Design review of the part built by this model. Coordinates are the model's own, in mm. A direction names the side the tool comes from. Coordinates: 2 decimals unless noted, no trailing zeros. Write each loop counter-clockwise with the first axis right and the second up, starting at its lowest first coordinate (ties: lowest second). Pieces come first, ordered by that corner, then holes. Notation, with made-up numbers: (-24, 32.25) - (7, 32.25) arc R5 cw to (7, 38.25) - close; hole circle Ø5 at (20.5, 20). An arc over 180 degrees is marked (long way). Answer as a JSON object with one key per item and string values.
```python
from build123d import *

# Parameters (mm, degrees)
SKETCH_2_W               = 50
SKETCH_2_H               = 30
SKETCH_2_W_2             = 48
SKETCH_2_H_2             = 28
EXTRUDE_1_DEPTH          = 150
SKETCH_3_R               = 1.525
CUT_EXTRUDE_1_DEPTH      = 10
PATTERN_LINEAR_1_COUNT   = 7
PATTERN_LINEAR_1_PITCH   = 30
SKETCH_4_R               = 1.525
CUT_EXTRUDE_2_DEPTH      = 10
PATTERN_LINEAR_2_COUNT   = 15
PATTERN_LINEAR_2_PITCH   = 20
CUT_EXTRUDE_3_DEPTH      = 10
PATTERN_LINEAR_3_COUNT   = 7
PATTERN_LINEAR_3_PITCH   = 40
SKETCH_6_R               = 4
CUT_EXTRUDE_4_DEPTH      = 10
PATTERN_LINEAR_4_COUNT   = 7
PATTERN_LINEAR_4_PITCH   = 30
SKETCH_7_R               = 1.525
CUT_EXTRUDE_5_DEPTH      = 90
SKETCH_8_R               = 1.525
CUT_EXTRUDE_6_DEPTH      = 10
SKETCH_10_R              = 1.525
CUT_EXTRUDE_7_DEPTH      = 51
SKETCH_12_R              = 1.525
CUT_EXTRUDE_9_DEPTH      = 1
CUT_EXTRUDE_9_DEPTH_BACK = 31
SKETCH_14_R              = 1.525
CUT_EXTRUDE_10_DEPTH     = 10


with BuildPart() as part:
    # 草图2 → 凸台-拉伸1 (new body, symmetric)
    with BuildSketch(Plane.XY):
        Rectangle(SKETCH_2_W, SKETCH_2_H)
        Rectangle(SKETCH_2_W_2, SKETCH_2_H_2, mode=Mode.SUBTRACT)
    extrude(amount=EXTRUDE_1_DEPTH, both=True)

    # 草图3 → 切除-拉伸1 (cut)
    with BuildSketch(Plane(origin=(25, 0, 0), x_dir=(0, 0, -1), z_dir=(1, 0, 0))):
        with Locations((-130, 5)):
            Circle(SKETCH_3_R)
    cut_extrude_1 = extrude(amount=-CUT_EXTRUDE_1_DEPTH, mode=Mode.SUBTRACT)

    # 阵列(线性)1: 切除-拉伸1 ×7
    with Locations(*[(0, 0, -i * PATTERN_LINEAR_1_PITCH) for i in range(1, PATTERN_LINEAR_1_COUNT)]):
        add(cut_extrude_1, mode=Mode.SUBTRACT)

    # 草图4 → 切除-拉伸2 (cut)
    with BuildSketch(Plane(origin=(0, 15, 0), x_dir=(1, 0, 0), z_dir=(0, 1, 0))):
        with Locations((-12, 140)):
            Circle(SKETCH_4_R)
        with Locations((12, 140)):
            Circle(SKETCH_4_R)
    cut_extrude_2 = extrude(amount=-CUT_EXTRUDE_2_DEPTH, mode=Mode.SUBTRACT)

    # 阵列(线性)2: 切除-拉伸2 ×15
    with Locations(*[(0, 0, i * PATTERN_LINEAR_2_PITCH) for i in range(1, PATTERN_LINEAR_2_COUNT)]):
        add(cut_extrude_2, mode=Mode.SUBTRACT)

    # 草图5 → 切除-拉伸3 (cut)
    with BuildSketch(Plane(origin=(0, -14, 0), x_dir=(1, 0, 0), z_dir=(0, 1, 0))):
        with BuildLine():
            Line((-17.5, -140), (-17.5, -120))
            ThreePointArc((-17.5, -120), (-12, -114.5), (-6.5, -120))
            Line((-6.5, -120), (-6.5, -140))
            ThreePointArc((-6.5, -140), (-12, -145.5), (-17.5, -140))
        make_face()
        with BuildLine():
            Line((17.5, -140), (17.5, -120))
            ThreePointArc((17.5, -120), (12, -114.5), (6.5, -120))
            Line((6.5, -120), (6.5, -140))
            ThreePointArc((6.5, -140), (12, -145.5), (17.5, -140))
        make_face()
    cut_extrude_3 = extrude(amount=-CUT_EXTRUDE_3_DEPTH, mode=Mode.SUBTRACT)

    # 阵列(线性)3: 切除-拉伸3 ×7
    with Locations(*[(0, 0, -i * PATTERN_LINEAR_3_PITCH) for i in range(1, PATTERN_LINEAR_3_COUNT)]):
        add(cut_extrude_3, mode=Mode.SUBTRACT)

    # 草图6 → 切除-拉伸4 (cut)
    with BuildSketch(Plane(origin=(-24, 0, 0), x_dir=(0, 0, -1), z_dir=(1, 0, 0))):
        with Locations((-130, 5)):
            Circle(SKETCH_6_R)
    cut_extrude_4 = extrude(amount=-CUT_EXTRUDE_4_DEPTH, mode=Mode.SUBTRACT)

    # 阵列(线性)4: 切除-拉伸4 ×7
    with Locations(*[(0, 0, -i * PATTERN_LINEAR_4_PITCH) for i in range(1, PATTERN_LINEAR_4_COUNT)]):
        add(cut_extrude_4, mode=Mode.SUBTRACT)

    # 草图7 → 切除-拉伸5 (cut)
    with BuildSketch(Plane.XZ.offset(15)):
        with Locations((-19, -144)):
            Circle(SKETCH_7_R)
        with Locations((1, -144)):
            Circle(SKETCH_7_R)
    extrude(amount=-CUT_EXTRUDE_5_DEPTH, mode=Mode.SUBTRACT)

    # 草图8 → 切除-拉伸6 (cut)
    with BuildSketch(Plane.XZ.offset(15)):
        with Locations((19, -10)):
            Circle(SKETCH_8_R)
        with Locations((-19, -10)):
            Circle(SKETCH_8_R)
        with Locations((-19, -90)):
            Circle(SKETCH_8_R)
        with Locations((19, -90)):
            Circle(SKETCH_8_R)
        with Locations((-19, 70)):
            Circle(SKETCH_8_R)
        with Locations((19, 70)):
            Circle(SKETCH_8_R)
    extrude(amount=-CUT_EXTRUDE_6_DEPTH, mode=Mode.SUBTRACT)

    # 草图10 → 切除-拉伸7 (cut, through all)
    with BuildSketch(Plane(origin=(25, 0, 0), x_dir=(0, 0, -1), z_dir=(1, 0, 0))):
        with Locations((139, -1)):
            Circle(SKETCH_10_R)
    extrude(amount=-CUT_EXTRUDE_7_DEPTH, mode=Mode.SUBTRACT)

    # 草图12 → 切除-拉伸9 (cut, two sides)
    with BuildSketch(Plane.XZ.offset(15)) as cut_extrude_9_sk:
        with Locations((1, -138.5)):
            Circle(SKETCH_12_R)
    extrude(amount=CUT_EXTRUDE_9_DEPTH, mode=Mode.SUBTRACT)
    extrude(cut_extrude_9_sk.sketch, amount=-CUT_EXTRUDE_9_DEPTH_BACK, mode=Mode.SUBTRACT)

    # 草图14 → 切除-拉伸10 (cut)
    with BuildSketch(Plane(origin=(25, 0, 0), x_dir=(0, 0, -1), z_dir=(1, 0, 0))):
        with Locations((143.5, -1)):
            Circle(SKETCH_14_R)
    extrude(amount=-CUT_EXTRUDE_10_DEPTH, mode=Mode.SUBTRACT)


solid = part.part
```
(1) For pin 1 (8 mm diameter, centred on x = -8, y = 8.5, fed in from -Z), flat-tipped, find the tip position at first contact; note if it passes through.
Solved:
{"pin 1": "passes through"}
(2) To check wall thickness, follow line 1 (X direction, y = 14.8, z = 120) (3 decimals); line 2 (Z direction, x = -19, y = -14.45) (3 decimals); line 3 (Y direction, x = 21, z = -110). State the ranges of each line that lie inside material, in increasing order. Write a range as from..to.
Solved:
{"line 1": "x = -25..-13.525, -10.475..10.475, 13.525..25", "line 2": "z = -150..-145.525, -142.475..-91.525, -88.475..-11.525, -8.475..68.475, 71.525..150", "line 3": "y = -15..-14, 14..15"}
(3) Tool access review of faces 4 (the face through (0, -15, 2)), 5 (the face through (11.9, -14.5, 145.5)), 6 (the face through (0, 15, 2)), 7 (the face through (0, -14, 2)), 8 (the face through (-24.493, 3.468, 66.305)): name each direction out of +Z, -Z, +X, -X, +Y, -Y from which nothing blocks a thin tool from reaching the whole face with its end or side.
Solved:
{"face 4": "+Z, -Z, +X, -X, -Y", "face 5": "-Y", "face 6": "+Z, -Z, +X, -X, +Y", "face 7": "+Z, -Z", "face 8": "-X"}
(4) Take a section at A-A, the plane y = -8. Write out the cut boundary in (x, z), and give its area (3 significant figures).
Solved:
{"outline": "(-25, -150) - (-24, -150) - (-24, 150) - (-25, 150) - close; (24, -150) - (25, -150) - (25, 150) - (24, 150) - close", "area": "600 mm^2"}
(5) The part is to be moulded in two halves that separate along Z. For faces 1 (the face through (-24.49, 7.7, -47.05)), 2 (the face through (-7.5, 14.5, 150)), 3 (the face through (24, 0, 2)), say which applies: pulls with the +Z half, pulls with the -Z half, needs draft (parallel to the pull), parting line crosses it, or undercut.
Solved:
{"face 1": "undercut", "face 2": "pulls with the +Z half", "face 3": "needs draft"}
